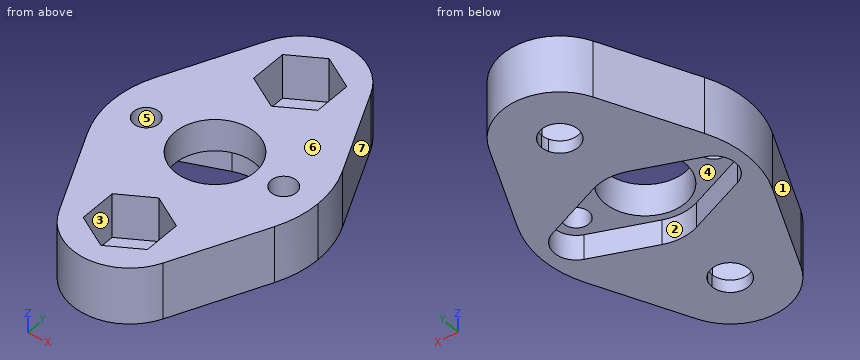
from build123d import *

# Parameters (mm, degrees)
F0_R     = 1.1
F0_R_2   = 3.5
F1_DEPTH = 5
F2_R     = 1.6
F3_DEPTH = 3.9
F5_START = -2.8
F5_DEPTH = 22.2


with BuildPart() as f1:
    # F0 (on Top) → F1 (new body)
    with BuildSketch(Plane.XY):
        with BuildLine():
            ThreePointArc((-1.4743268336, 8.8784210526), (-0.3170781184, 11.0682670266), (1.6, 9.5))
            ThreePointArc((1.6, 9.5), (1.5682670266, 9.1829218816), (1.4743268336, 8.8784210526))
            ThreePointArc((1.4743268336, 8.8784210526), (3.1253325319, 8.4399227819), (4.6637452107, 7.6973684211))
            ThreePointArc((4.6637452107, 7.6973684211), (4.9152174954, 8.5831374295), (5, 9.5))
            ThreePointArc((5, 9.5), (4.882412579, 10.5779830278), (4.5351810367, 11.6052631579))
            ThreePointArc((4.5351810367, 11.6052631579), (0, 14.5), (-4.5351810367, 11.6052631579))
            ThreePointArc((-4.5351810367, 11.6052631579), (-4.9972964036, 9.6644039381), (-4.6637452107, 7.6973684211))
            ThreePointArc((-4.6637452107, 7.6973684211), (-3.1253325319, 8.4399227819), (-1.4743268336, 8.8784210526))
        make_face()
        with BuildLine():
            ThreePointArc((1.4743268336, 8.8784210526), (0, 7.9), (-1.4743268336, 8.8784210526))
            ThreePointArc((-1.4743268336, 8.8784210526), (-3.1253325319, 8.4399227819), (-4.6637452107, 7.6973684211))
            ThreePointArc((-4.6637452107, 7.6973684211), (0, 4.5), (4.6637452107, 7.6973684211))
            ThreePointArc((4.6637452107, 7.6973684211), (3.1253325319, 8.4399227819), (1.4743268336, 8.8784210526))
        make_face()
        with BuildLine():
            ThreePointArc((4.6637452107, 7.6973684211), (0, 4.5), (-4.6637452107, 7.6973684211))
            ThreePointArc((-4.6637452107, 7.6973684211), (-6.7045766773, 6.0040529294), (-8.1633258661, 3.7894736842))
            ThreePointArc((-8.1633258661, 3.7894736842), (-9, 0), (-8.1633258661, -3.7894736842))
            ThreePointArc((-8.1633258661, -3.7894736842), (-6.7045766773, -6.0040529294), (-4.6637452107, -7.6973684211))
            ThreePointArc((-4.6637452107, -7.6973684211), (0, -4.5), (4.6637452107, -7.6973684211))
            ThreePointArc((4.6637452107, -7.6973684211), (6.7045766773, -6.0040529294), (8.1633258661, -3.7894736842))
            ThreePointArc((8.1633258661, -3.7894736842), (8.7883426423, -1.94036945), (9, 0))
            ThreePointArc((9, 0), (8.7883426423, 1.94036945), (8.1633258661, 3.7894736842))
            ThreePointArc((8.1633258661, 3.7894736842), (6.7045766773, 6.0040529294), (4.6637452107, 7.6973684211))
        make_face()
        with Locations((-6, 0)):
            Circle(F0_R, mode=Mode.SUBTRACT)
        Circle(F0_R_2, mode=Mode.SUBTRACT)
        with Locations((6, 0)):
            Circle(F0_R, mode=Mode.SUBTRACT)
        with BuildLine():
            ThreePointArc((-8.1633258661, 3.7894736842), (-6.7045766773, 6.0040529294), (-4.6637452107, 7.6973684211))
            ThreePointArc((-4.6637452107, 7.6973684211), (-4.9972964036, 9.6644039381), (-4.5351810367, 11.6052631579))
            Line((-4.5351810367, 11.6052631579), (-8.1633258661, 3.7894736842))
        make_face()
        with BuildLine():
            ThreePointArc((5, 9.5), (4.9152174954, 8.5831374295), (4.6637452107, 7.6973684211))
            ThreePointArc((4.6637452107, 7.6973684211), (6.7045766773, 6.0040529294), (8.1633258661, 3.7894736842))
            Line((8.1633258661, 3.7894736842), (4.5351810367, 11.6052631579))
            ThreePointArc((4.5351810367, 11.6052631579), (4.882412579, 10.5779830278), (5, 9.5))
        make_face()
        with BuildLine():
            ThreePointArc((-4.6637452107, -7.6973684211), (-6.7045766773, -6.0040529294), (-8.1633258661, -3.7894736842))
            Line((-8.1633258661, -3.7894736842), (-4.5351810367, -11.6052631579))
            ThreePointArc((-4.5351810367, -11.6052631579), (-4.9972964036, -9.6644039381), (-4.6637452107, -7.6973684211))
        make_face()
        with BuildLine():
            ThreePointArc((-1.4743268336, -8.8784210526), (-3.1253325319, -8.4399227819), (-4.6637452107, -7.6973684211))
            ThreePointArc((-4.6637452107, -7.6973684211), (-4.9972964036, -9.6644039381), (-4.5351810367, -11.6052631579))
            ThreePointArc((-4.5351810367, -11.6052631579), (0, -14.5), (4.5351810367, -11.6052631579))
            ThreePointArc((4.5351810367, -11.6052631579), (4.882412579, -10.5779830278), (5, -9.5))
            ThreePointArc((5, -9.5), (4.9152174954, -8.5831374295), (4.6637452107, -7.6973684211))
            ThreePointArc((4.6637452107, -7.6973684211), (3.1253325319, -8.4399227819), (1.4743268336, -8.8784210526))
            ThreePointArc((1.4743268336, -8.8784210526), (1.5682670266, -9.1829218816), (1.6, -9.5))
            ThreePointArc((1.6, -9.5), (-0.3170781184, -11.0682670266), (-1.4743268336, -8.8784210526))
        make_face()
        with BuildLine():
            ThreePointArc((4.6637452107, -7.6973684211), (0, -4.5), (-4.6637452107, -7.6973684211))
            ThreePointArc((-4.6637452107, -7.6973684211), (-3.1253325319, -8.4399227819), (-1.4743268336, -8.8784210526))
            ThreePointArc((-1.4743268336, -8.8784210526), (0, -7.9), (1.4743268336, -8.8784210526))
            ThreePointArc((1.4743268336, -8.8784210526), (3.1253325319, -8.4399227819), (4.6637452107, -7.6973684211))
        make_face()
        with BuildLine():
            Line((4.5351810367, -11.6052631579), (8.1633258661, -3.7894736842))
            ThreePointArc((8.1633258661, -3.7894736842), (6.7045766773, -6.0040529294), (4.6637452107, -7.6973684211))
            ThreePointArc((4.6637452107, -7.6973684211), (4.9152174954, -8.5831374295), (5, -9.5))
            ThreePointArc((5, -9.5), (4.882412579, -10.5779830278), (4.5351810367, -11.6052631579))
        make_face()
    extrude(amount=F1_DEPTH)

    # F2 (on face) → F3 (cut)
    with BuildSketch(Plane.XY.offset(5)):
        Polygon((2.8, 7.8834192463), (2.8, 11.1165807537), (0, 12.7331615075), (-2.8, 11.1165807537), (-2.8, 7.8834192463), (0, 6.2668384925), align=None)
        with Locations((0, 9.5)):
            Circle(F2_R, mode=Mode.SUBTRACT)
        Polygon((-2.8, -11.1165807537), (0, -12.7331615075), (2.8, -11.1165807537), (2.8, -7.8834192463), (0, -6.2668384925), (-2.8, -7.8834192463), align=None)
    extrude(amount=-F3_DEPTH, mode=Mode.SUBTRACT)

    # F4 (on face) → F5 (cut)
    with BuildSketch(Plane.XY.offset(5).offset(F5_START)):
        with BuildLine():
            Line((-1.5033333333, 3.8144447681), (-6.6966666667, 1.7676695267))
            ThreePointArc((-6.6966666667, 1.7676695267), (-7.9, 0), (-6.6966666667, -1.7676695267))
            Line((-6.6966666667, -1.7676695267), (-1.5033333333, -3.8144447681))
            ThreePointArc((-1.5033333333, -3.8144447681), (0, -4.1), (1.5033333333, -3.8144447681))
            Line((1.5033333333, -3.8144447681), (6.6966666667, -1.7676695267))
            ThreePointArc((6.6966666667, -1.7676695267), (7.9, 0), (6.6966666667, 1.7676695267))
            Line((6.6966666667, 1.7676695267), (1.5033333333, 3.8144447681))
            ThreePointArc((1.5033333333, 3.8144447681), (0, 4.1), (-1.5033333333, 3.8144447681))
        make_face()
    extrude(amount=-F5_DEPTH, mode=Mode.SUBTRACT)


solid = f1.part
Design review of the part built by this model. Coordinates are the model's own, in mm. Face numbers are marked on the shaded views. A direction names the side the tool comes from. Coordinates: 2 decimals unless noted, no trailing zeros. Loops run counter-clockwise (first coordinate to the right, second up) from the corner with the lowest first, then second, coordinate; pieces in that order, holes last. Notation, with made-up numbers: (-4.5, 14.25) - (40.5, 14.25) arc R23 ccw to (40.5, 37.25) - close; hole circle Ø11 at (11.25, -26). An arc over 180 degrees is marked (long way). Use CSV: the item, a comma, the result in double quotes. Start each with the question number.
1. Add section D-D on y = 3. Give the boundary of the cut face in (x, z), plus the area to 4 significant figures.
2. To check wall thickness, follow probe 1 along X at (y, z) = (0, 3.95); probe 2 along Y at (x, z) = (1, 1.2); probe 3 along Y at (x, z) = (0.25, 1.2). State the ranges of each line that lie inside material, in increasing order.
3. For the marked faces 1, 2 and 3, list the 3-axis set-ups (+Z, -Z, +X, -X, +Y, -Y) from which the entire face can be reached by the end or side of a thin tool; tool diameter is ignored.
4. Add section B-B on x = 6. Give the boundary of the cut face in (y, z).
5. Add section A-A on z = 1.75. Give the boundary of the cut face in (x, y).
6. Clearance check with flat-ended pins moving along their axes: pin 1 (6.5 mm diameter, centred on x = 0, y = 0, fed in from +Z); pin 2 (1 mm diameter, centred on y = 8.5, z = 4, fed in from +X); pin 3 (1.5 mm diameter, centred on y = -11, z = 3.5, fed in from -X); pin 4 (2.5 mm diameter, centred on y = -10, z = 3.5, fed in from -X). State where each tip first meets the part, or that it passes through.
7. Mouldability with a two-part tool opening along Y and no side actions: class the marked faces 4, 5, 6 and 7 as released by +Y, released by -Y, zero draft, split by the parting line, or undercut.
8. Add section C-C on z = 3.9. Give the boundary of the cut face in (x, y), plus the area to 3 significant figures.
Resolved:
1,outline,"(-8.49, 0) - (-3.57, 0) - (-3.57, 2.2) - (-1.8, 2.2) - (-1.8, 5) - (-8.49, 5) - close; (1.8, 2.2) - (3.57, 2.2) - (3.57, 0) - (8.49, 0) - (8.49, 5) - (1.8, 5) - close"
1,area,"59.05 mm2"
2,probe 1,"-9 to -7.1, -4.9 to -3.5, 3.5 to 4.9, 7.1 to 9"
2,probe 2,"-14.4 to -12.16, -6.84 to -3.98, 3.98 to 6.84, 12.16 to 14.4"
2,probe 3,"-14.49 to -12.59, -6.41 to -4.09, 4.09 to 6.41, 12.59 to 14.49"
3,face 1,"+Z, -Z, -X, -Y"
3,face 2,"-Z"
3,face 3,"+Z"
4,outline,"(-8.45, 0) - (-2.04, 0) - (-2.04, 2.2) - (-1.1, 2.2) - (-1.1, 5) - (-8.45, 5) - close; (1.1, 2.2) - (2.04, 2.2) - (2.04, 0) - (8.45, 0) - (8.45, 5) - (1.1, 5) - close"
5,outline,"(-8.16, -3.79) - (-4.54, -11.61) arc R5 ccw to (4.54, -11.61) - (8.16, -3.79) arc R9 ccw to (8.16, 3.79) - (4.54, 11.61) arc R5 ccw to (-4.54, 11.61) - (-8.16, 3.79) arc R9 ccw to start; hole (-6.7, -1.77) - (-1.5, -3.81) arc R4.1 ccw to (1.5, -3.81) - (6.7, -1.77) arc R1.9 ccw to (6.7, 1.77) - (1.5, 3.81) arc R4.1 ccw to (-1.5, 3.81) - (-6.7, 1.77) arc R1.9 ccw to start; hole (-2.8, -11.12) - (0, -12.73) - (2.8, -11.12) - (2.8, -7.88) - (0, -6.27) - (-2.8, -7.88) - close; hole (-2.8, 7.88) - (0, 6.27) - (2.8, 7.88) - (2.8, 11.12) - (0, 12.73) - (-2.8, 11.12) - close"
6,pin 1,"through"
6,pin 2,"x = 6.21"
6,pin 3,"x = -5.16"
6,pin 4,"x = -5.86"
7,face 4,"undercut"
7,face 5,"undercut"
7,face 6,"zero draft"
7,face 7,"released by +Y"
8,outline,"(-8.16, -3.79) - (-4.54, -11.61) arc R5 ccw to (4.54, -11.61) - (8.16, -3.79) arc R9 ccw to (8.16, 3.79) - (4.54, 11.61) arc R5 ccw to (-4.54, 11.61) - (-8.16, 3.79) arc R9 ccw to start; hole circle Ø2.2 at (-6, 0); hole circle Ø7 at (0, 0); hole (-2.8, -11.12) - (0, -12.73) - (2.8, -11.12) - (2.8, -7.88) - (0, -6.27) - (-2.8, -7.88) - close; hole (-2.8, 7.88) - (0, 6.27) - (2.8, 7.88) - (2.8, 11.12) - (0, 12.73) - (-2.8, 11.12) - close; hole circle Ø2.2 at (6, 0)"
8,area,"268 mm2"
